```python
from build123d import *

# Parameters (mm, degrees)
F4_W     = 24
F4_H     = 14
F5_DEPTH = 9
F6_W     = 20
F6_H     = 10
F7_DEPTH = 5
F8_R     = 1


with BuildPart() as f5:
    # F4 (on Front) → F5 (new body)
    with BuildSketch(Plane.XZ):
        with Locations((0, 7)):
            Rectangle(F4_W, F4_H)
    extrude(amount=F5_DEPTH)

    # F6 (on face) → F7 (cut)
    with BuildSketch(Plane.XZ.offset(9)):
        with Locations((0, 7)):
            Rectangle(F6_W, F6_H)
    extrude(amount=-F7_DEPTH, mode=Mode.SUBTRACT)

    # F8
    f8_edges = [f5.edges().sort_by_distance(p)[0] for p in [
        (-12, -4.5, 14),
        (12, -4.5, 14),
        (-10, -6.5, 12),
        (10, -6.5, 12),
        (10, -6.5, 2),
        (-10, -6.5, 2),
    ]]
    fillet(f8_edges, radius=F8_R)


solid = f5.part
```
Geometry check sheet. Reference: the model listing, model coordinates, mm. A direction names the side the tool comes from. Round coordinates to 2 decimals unless told otherwise and drop trailing zeros. Loops run counter-clockwise (first coordinate to the right, second up) from the corner with the lowest first, then second, coordinate; pieces in that order, holes last. Notation, with made-up numbers: M -4,29.5 L 28,29.5 A24 ccw 28,40.5 Z; hole C -24.75,81 d2. An arc over 180 degrees is marked long. Return JSON: item names as keys, results as strings. Group by question number.
(1) Section check B-B, the plane z = 5.25. Enter the section's corners in (x, y), and give its area (3 significant figures).
(2) Section check A-A, the plane y = -6.75. Enter the section's corners in (x, z), and give its area (3 significant figures).
(3) Mould release check, pull along X, two halves, no side actions. Record for faces 3 (the face through (11.699, -4.563, 13.715)), 4 (the face through (-11.715, -4.563, 13.699)), 5 (the face through (9.699, -6.465, 2.285)): pulls with the +X half, pulls with the -X half, needs draft (parallel to the pull), parting line crosses it, or undercut.
(4) Set-up check for faces 1 (the face through (-9.699, -6.465, 2.285)), 2 (the face through (0, 0, 7)): record each of +Z, -Z, +X, -X, +Y, -Y from which the full face is reachable in a straight line by a thin tool's end or side.
(5) Scan lines: line 1 along Z through (x, y) = (2.75, -4.5); line 2 along X through (y, z) = (-5.25, 10); line 3 along Y through (x, z) = (1.75, 5). Record each from-to range of solid material in increasing order. Write a range as [from, to].
(6) Section check C-C, the plane x = 5.5. Enter the section's corners in (y, z), and give its area (3 significant figures).
(7) Go/stop test with a flat-tipped pin: pin 1 (1 mm diameter, centred on x = 2, z = 9.5, fed in from -Y). Record where the tip stops, or that it passes through.
Data:
{
 "1": {"outline": "M -12,-9 L -10,-9 L -10,-4 L 10,-4 L 10,-9 L 12,-9 L 12,0 L -12,0 Z", "area": "116 mm²"},
 "2": {"outline": "M -12,0 L 12,0 L 12,13 A1 ccw 11,14 L -11,14 A1 ccw -12,13 Z; hole M -10,3 A1 ccw -9,2 L 9,2 A1 ccw 10,3 L 10,11 A1 ccw 9,12 L -9,12 A1 ccw -10,11 Z", "area": "136 mm²"},
 "3": {"face 3": "pulls with the +X half", "face 4": "pulls with the -X half", "face 5": "undercut"},
 "4": {"face 1": "-Y", "face 2": "+Z, -Z, +X, -X, +Y"},
 "5": {"line 1": "[0, 2], [12, 14]", "line 2": "[-12, -10], [10, 12]", "line 3": "[-4, 0]"},
 "6": {"outline": "M -9,0 L 0,0 L 0,14 L -9,14 L -9,12 L -4,12 L -4,2 L -9,2 Z", "area": "76.0 mm²"},
 "7": {"pin 1": "y = -4"}
}
